Autodesk Inventor part; units mm, degrees
ref_plane "YZ Plane" through (0, 0, 0) normal (1, 0, 0) x (0, 1, 0)
ref_plane "XZ Plane" through (0, 0, 0) normal (0, 1, 0) x (-1, 0, 0)
ref_plane "XY Plane" through (0, 0, 0) normal (0, 0, 1) x (1, 0, 0)
sketch "スケッチ1" plane through (0, 0, 0) normal (1, 0, 0) x (0, 1, 0)
  circle A0 centre (0, 0) radius 30
  line L0 (10, -28.2843) -> (10, -43)
  line L1 (10, -43) -> (-10, -43)
  line L2 (-10, -43) -> (-10, -28.2843)
  line L3 (10, -43) -> (25.9808, -15)
  line L4 (-10, -43) -> (-25.9808, -15)
  circle A1 centre (0, 0) radius 2.35
  circle A2 centre (0, 0) radius 28
  point P0 (0, -30)
  point P1 (0, -28.05)
  point P2 (0, -26.4333)
  dimension "d2" = 20
  dimension "d10" = 4.7
  dimension "d34" = 13
  dimension "d39" = 2
extrude "押し出し8" add sketch "スケッチ1" along normal blind 10 contours A0 | A0 L2 L4 | L3 L0 A0 | A0 L0 L1 L2 | A2
extrude "押し出し9" cut sketch "スケッチ1" along normal blind 3 contours A2
sketch "スケッチ3" plane through (0, 0, 0) normal (-1, 0, 0) x (0, 0, 1)
  line L0 (-15.35, 6.25) -> (-38, 6.25)
  line L1 (-38, 6.25) -> (-38, -6.25)
  line L2 (-38, -6.25) -> (-15.35, -6.25)
  line L3 (-15.35, -6.25) -> (-15.35, 6.25)
  line L4 (-15.35, 6.25) -> (-38, -6.25) construction
  line L5 (-38, 6.25) -> (-15.35, -6.25) construction
  line L6 (-15.35, -6.25) -> (-10.35, -6.25)
  line L7 (-10.35, -6.25) -> (-10.35, 6.25)
  line L8 (-10.35, 6.25) -> (-15.35, 6.25)
  line L9 (-15.35, 6.25) -> (-15.35, -6.25)
  line L10 (-38, -6.25) -> (-43, -6.25)
  line L11 (-43, -6.25) -> (-43, 6.25)
  line L12 (-43, 6.25) -> (-38, 6.25)
  line L13 (-38, 6.25) -> (-38, -6.25)
  circle A0 centre (-31.75, 0) radius 6.25
  circle A1 centre (-31.75, 0) radius 2.4
  line L14 (-43, -10) -> (-43, 10)
  point P0 (0, 0)
  point P1 (-26.675, 0)
  dimension "d42" = 22.65
  dimension "d43" = 12.5
  dimension "d44" = 5
  dimension "d45" = 5
  dimension "d46" = 12.5
  dimension "d47" = 0
  dimension "d48" = 4.8
  dimension "d49" = 0
  dimension "d50" = 0
extrude "押し出し10" cut sketch "スケッチ3" against normal blind 10 contours A0
extrude "押し出し11" cut sketch "スケッチ3" against normal blind 10 contours A1
extrude "押し出し12" cut sketch "スケッチ3" against normal blind 6 contours L3 L2 A0 L0 | A0 L1 L0 | A0 L2 L1
extrude "押し出し13" cut sketch "スケッチ3" against normal blind 3 contours L1 L10 L11 L12
sketch "スケッチ5" plane through (10, 0, 0) normal (1, 0, 0) x (0, 0, -1)
  arc A0 (31.75, 6.25) -> (31.75, -6.25) centre (31.75, 0) ccw
  line L0 (25.8286, -2) -> (20.8286, -2)
  line L1 (20.8286, -2) -> (20.8286, 2)
  line L2 (20.8286, 2) -> (25.8286, 2)
  line L3 (25.8286, 2) -> (25.8286, -2)
  point P0 (0, 0)
  dimension "d63" = 4
  dimension "d64" = 2
  dimension "d65" = 5
extrude "押し出し14" cut sketch "スケッチ5" against normal blind 10
sketch "スケッチ6" plane through (10, 0, 0) normal (1, 0, 0) x (0, 0, -1)
  circle A0 centre (38, -8) radius 1.5
  circle A1 centre (38, 8) radius 1.5
  line L0 (43, -10) -> (43, 10)
  circle A2 centre (33, -8) radius 1.5
  circle A3 centre (33, 8) radius 1.5
  point P0 (0, 0)
  dimension "d68" = 5
  dimension "d69" = 5
  dimension "d74" = 3
  dimension "d76" = 16
  dimension "d77" = 2
  dimension "d78" = 2
  dimension "d81" = 3
  dimension "d82" = 5
  dimension "d83" = 5
  dimension "d84" = 3
extrude "押し出し15" cut sketch "スケッチ6" against normal blind 100 contours A0 | A1
extrude "押し出し16" cut sketch "スケッチ6" against normal blind 100 contours A2 | A3
properties part number "BasePart"
Build history of the part. All positions in model axes, mm. A direction names the side the tool comes from. Round coordinates to 2 decimals unless told otherwise and drop trailing zeros. Write each loop counter-clockwise with the first axis right and the second up, starting at its lowest first coordinate (ties: lowest second). Pieces come first, ordered by that corner, then holes. Notation, with made-up numbers: (-26, -4) - (21, -4) arc R15 ccw to (21, 9) - close; hole circle Ø6 at (33.25, 71). An arc over 180 degrees is marked (long way). One line per question, with ' | ' between items.
1. Band-saw the part on C-C, the plane x = 8.75. Write the cut outline in (y, z).
Results are:
outline: (-25.98, -15) - (-10, -43) - (10, -43) - (25.98, -15) arc R30 ccw (long way) to start; hole circle Ø3 at (-8, -38); hole circle Ø3 at (-8, -33); hole circle Ø4.7 at (0, 0); hole (-2, -25.83) arc R6.25 ccw (long way) to (2, -25.83) - (2, -20.83) - (-2, -20.83) - close; hole circle Ø3 at (8, -38); hole circle Ø3 at (8, -33)
2. Band-saw the part on B-B, the plane z = 24.5. Write the cut outline in (x, y).
Results are:
outline: (0, -17.31) - (10, -17.31) - (10, 17.31) - (0, 17.31) - (0, 13.56) - (3, 13.56) - (3, -13.56) - (0, -13.56) - close
3. Drill centre lines: line 1 along Y through (x, z) = (6.5, -33); line 2 along Z through (x, y) = (7.25, 0); line 3 along Y through (x, z) = (7.3, -31.75). Where is each one in solid material? Low to high. Write a range as from..to.
Results are:
line 1: -15.71..-9.5, -6.5..-6.12, 6.12..6.5, 9.5..15.71 | line 2: -43..-38, -20.83..-2.35, 2.35..30 | line 3: -16.42..-8.83, -7.17..-6.25, 6.25..7.17, 8.83..16.42
4. Band-saw the part on A-A, the plane y = -8. Write the cut outline in (x, z), and give its area (3 significant figures).
Results are:
outline: (0, -43) - (10, -43) - (10, -39.5) - (0, -39.5) - close; (0, -36.5) - (10, -36.5) - (10, -34.5) - (0, -34.5) - close; (0, -31.5) - (10, -31.5) - (10, 28.91) - (0, 28.91) - (0, 26.83) - (3, 26.83) - (3, -26.83) - (0, -26.83) - close | area: 498 mm^2
5. Mould opens along Z. For faces 6 (the face through (4.93, -17.879, -29.196)), 7 (the face through (4, 0, -38)), 8 (the face through (6, 0, -20)), 9 (the face through (0, -7, -28)) say: released by +Z, released by -Z, zero draft, split by the parting line, or undercut.
Results are:
face 6: released by -Z | face 7: undercut | face 8: undercut | face 9: zero draft
6. Drop flat-ended pins along their axis: pin 1 Ø3 at (x, z) = (2.5, -35) entering from -Y; pin 2 Ø5 at (x, z) = (2, -27.5) entering from -Y; pin 3 Ø4.5 at (x, z) = (8, -23.5) entering from +Y. Give the stop position or say it passes through.
Results are:
pin 1: y = -15.42 | pin 2: y = -20.27 | pin 3: y = 22.41
7. Band-saw the part on D-D, the plane y = 22. Write the cut outline in (x, z).
Results are:
outline: (0, -21.97) - (10, -21.97) - (10, 20.4) - (0, 20.4) - (0, 17.32) - (3, 17.32) - (3, -17.32) - (0, -17.32) - close
8. Tool access for faces 1 (the face through (6, 0, -43)), 2 (the face through (4.93, 17.879, -29.196)), 3 (the face through (3, 0, -41)), 4 (the face through (8, 0, -20.829)), 5 (the face through (6, 5, -37)): list every direction of +Z, -Z, +X, -X, +Y, -Y with a clear straight run to the whole face (end or side of a thin tool).
Results are:
face 1: -Z, +X, -X, +Y, -Y | face 2: -Z, +X, -X, +Y | face 3: -Z, -X | face 4: +X, -X | face 5: -X
